The listing builds one solid part. Answer for the finished solid, in the listing's coordinates (mm). Face numbers are marked on the shaded views. Give positions to 0.01 mm unless a question says otherwise; leave off trailing zeros. Loops run counter-clockwise (first coordinate to the right, second up) from the corner with the lowest first, then second, coordinate; pieces in that order, holes last. Notation, with made-up numbers: (-11, -29.5) -> (29, -29.5) arc R18 ccw to (29, -7.5) -> close; hole circle Ø1 at (66, 78). An arc over 180 degrees is marked (long way). One line per question, with ' | ' between items. Start each with the question number.
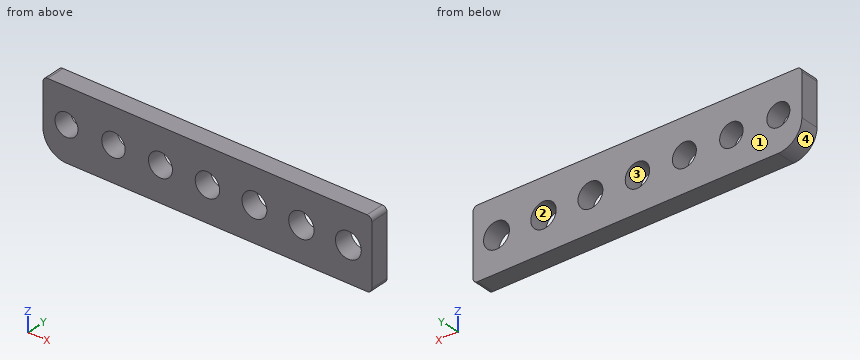
from build123d import *

# Parameters (mm, degrees)
SKETCH1_W           = 70
SKETCH1_H           = 15
SKETCH1_R           = 2.45
SKETCH1_R_2         = 2.5
SKETCH1_R_3         = 2.55
SKETCH1_R_4         = 2.6
SKETCH1_R_5         = 2.65
SKETCH1_R_6         = 2.7
SKETCH1_R_7         = 2.75
BOSS_EXTRUDE1_DEPTH = 4
FILLET1_R           = 5
FILLET2_R           = 1


with BuildPart() as part:
    # Sketch1 → Boss-Extrude1 (new body)
    with BuildSketch(Plane(origin=(0, 0, 0), x_dir=(1, 0, 0), z_dir=(0, 1, 0))):
        Rectangle(SKETCH1_W, SKETCH1_H)
        with Locations(Location((-30, 0, 0), (0, 0, 270))):
            Circle(SKETCH1_R, mode=Mode.SUBTRACT)
        with Locations(Location((-20, 0, 0), (0, 0, 270))):
            Circle(SKETCH1_R_2, mode=Mode.SUBTRACT)
        with Locations(Location((-10, 0, 0), (0, 0, 270))):
            Circle(SKETCH1_R_3, mode=Mode.SUBTRACT)
        with Locations(Location((0, 0, 0), (0, 0, 270))):
            Circle(SKETCH1_R_4, mode=Mode.SUBTRACT)
        with Locations(Location((10, 0, 0), (0, 0, 270))):
            Circle(SKETCH1_R_5, mode=Mode.SUBTRACT)
        with Locations(Location((20, 0, 0), (0, 0, 270))):
            Circle(SKETCH1_R_6, mode=Mode.SUBTRACT)
        with Locations(Location((30, 0, 0), (0, 0, 270))):
            Circle(SKETCH1_R_7, mode=Mode.SUBTRACT)
    extrude(amount=BOSS_EXTRUDE1_DEPTH)

    # Fillet1
    fillet1_edges = [part.edges().sort_by_distance(p)[0] for p in [
        (-35, 2, -7.5),
    ]]
    fillet(fillet1_edges, radius=FILLET1_R)

    # Fillet2
    fillet2_edges = [part.edges().sort_by_distance(p)[0] for p in [
        (35, 2, 7.5),
        (-35, 2, 7.5),
        (35, 2, -7.5),
    ]]
    fillet(fillet2_edges, radius=FILLET2_R)


solid = part.part
1. Straight lines are drawn through the part: L1, parallel to Z at x = 31, y = 1.8; L2, parallel to X at y = 3.8, z = -5.5; L3, parallel to Z at x = -22, y = 1.55. For each, find the intervals that lie inside material, in ascending order.
2. The part is cut by section B-B (z = -0.25). Count the separate pieces of the cut face and the enclosed holes in it, plus the area to 3 significant figures.
3. The part is cut by section C-C (y = 2.3). Write down the section's boundary in (x, z), plus the area to 3 significant figures.
4. The part is cut by section A-A (x = 0). Write down the section's boundary in (y, z).
5. The part is cut by section D-D (x = 30). Write down the section's boundary in (y, z), plus the area to 3 significant figures.
6. Determine the mould class of the marked faces 1, 2, 3 and 4 for opening direction Z: released by +Z, released by -Z, zero draft, split by the parting line, or undercut.
Check sheet entries:
1) L1: z = -7.5 to -2.56, 2.56 to 7.5 | L2: x = -34 to 35 | L3: z = -7.5 to -1.5, 1.5 to 7.5
2) separate pieces: 8 | enclosed holes: 0 | area: 135 mm^2
3) outline: (-35, -2.5) arc R5 ccw to (-30, -7.5) -> (34, -7.5) arc R1 ccw to (35, -6.5) -> (35, 6.5) arc R1 ccw to (34, 7.5) -> (-34, 7.5) arc R1 ccw to (-35, 6.5) -> close; hole circle Ø4.9 at (-30, 0); hole circle Ø5 at (-20, 0); hole circle Ø5.1 at (-10, 0); hole circle Ø5.2 at (0, 0); hole circle Ø5.3 at (10, 0); hole circle Ø5.4 at (20, 0); hole circle Ø5.5 at (30, 0) | area: 895 mm^2
4) outline: (0, -7.5) -> (4, -7.5) -> (4, -2.6) -> (0, -2.6) -> close; (0, 2.6) -> (4, 2.6) -> (4, 7.5) -> (0, 7.5) -> close
5) outline: (0, -7.5) -> (4, -7.5) -> (4, -2.75) -> (0, -2.75) -> close; (0, 2.75) -> (4, 2.75) -> (4, 7.5) -> (0, 7.5) -> close | area: 38.0 mm^2
6) face 1: zero draft | face 2: undercut | face 3: undercut | face 4: released by -Z
